```python
from build123d import *

# Parameters (mm, degrees)
SKETCH1_W           = 30
SKETCH1_H           = 13
BOSS_EXTRUDE1_DEPTH = 85
SKETCH2_W           = 22
SKETCH2_H           = 9
CUT_EXTRUDE2_DEPTH  = 85
SKETCH5_W           = 30
SKETCH5_H           = 13
BOSS_EXTRUDE3_DEPTH = 4
SKETCH12_W          = 22
SKETCH12_H          = 7
CUT_EXTRUDE4_DEPTH  = 13
SKETCH13_W          = 3
SKETCH13_H          = 80
CUT_EXTRUDE5_DEPTH  = 92.07140056


with BuildPart() as part:
    # Sketch1 → Boss-Extrude1 (new body)
    with BuildSketch(Plane(origin=(0, 0, 0), x_dir=(1, 0, 0), z_dir=(0, 1, 0))):
        with Locations((15, -6.5)):
            Rectangle(SKETCH1_W, SKETCH1_H)
    extrude(amount=BOSS_EXTRUDE1_DEPTH)

    # Sketch2 → Cut-Extrude2 (cut)
    with BuildSketch(Plane(origin=(0, 85, 0), x_dir=(1, 0, 0), z_dir=(0, 1, 0))):
        with Locations((15, -6.5)):
            Rectangle(SKETCH2_W, SKETCH2_H)
    extrude(amount=-CUT_EXTRUDE2_DEPTH, mode=Mode.SUBTRACT)

    # Sketch5 → Boss-Extrude3 (add)
    with BuildSketch(Plane(origin=(0, 0, 0), x_dir=(1, 0, 0), z_dir=(0, 1, 0))):
        with Locations((15, -6.5)):
            Rectangle(SKETCH5_W, SKETCH5_H)
    extrude(amount=-BOSS_EXTRUDE3_DEPTH)

    # Sketch12 → Cut-Extrude4 (cut)
    with BuildSketch(Plane.XY.offset(13)):
        with Locations((15, 3.5)):
            Rectangle(SKETCH12_W, SKETCH12_H)
    extrude(amount=-CUT_EXTRUDE4_DEPTH, mode=Mode.SUBTRACT)

    # Sketch13 → Cut-Extrude5 (cut, through all)
    with BuildSketch(Plane.ZY):
        with Locations((6.5, 40)):
            Rectangle(SKETCH13_W, SKETCH13_H)
    extrude(amount=-CUT_EXTRUDE5_DEPTH, mode=Mode.SUBTRACT)


solid = part.part
```
The model under review builds one solid part; all positions refer to its coordinate system, in mm. A direction names the side the tool comes from. Give positions to 0.01 mm unless a question says otherwise; leave off trailing zeros. Order: outer loops, then holes, each group sorted by start corner. A loop starts at its lowest first (then second) coordinate and runs counter-clockwise, first axis right, second up. Notation, with made-up numbers: (33, 83.25) - (52, 83.25) arc R18 ccw to (52, 115.25) - close; hole circle Ø3 at (81, -17.5). An arc over 180 degrees is marked (long way). Use CSV: the item, a comma, the result in double quotes. Start each with the question number.
Q1. We need section B-B, the plane x = 21.25. Write out the cut boundary in (y, z).
Q2. The part is to be moulded in two halves that separate along X. For faces 1 (the flat face through (0, 41, 9)), 2 (the flat face through (28, 39, 8)), 3 (the flat face through (15, 7, 1)), say which applies: +X half, -X half, draft (parallel to the pull), parting line (faces both ways), or undercut.
Q3. We need section C-C, the plane y = 16. Write out the cut boundary in (x, z), and give its area (3 significant figures).
Q4. To check wall thickness, follow line 1 along Y through (x, z) = (1.75, 7); line 2 along X through (y, z) = (25, 10.75); line 3 along Z through (x, y) = (26.75, 77). State the ranges of each line that lie inside material, in increasing order. Write a range as [from, to].
Q5. Tool access review of faces 4 (the flat face through (15, 47, 2)), 5 (the flat face through (28, 39, 5)), 6 (the flat face through (30, 41, 9)): name each direction out of +Z, -Z, +X, -X, +Y, -Y from which nothing blocks a thin tool from reaching the whole face with its end or side.
Q6. We need section A-A, the plane y = 5.5. Write out the cut boundary in (x, z), and give its area (3 significant figures).
Q7. We need section D-D, the plane z = 6.75. Write out the cut boundary in (x, y), and give its area (3 significant figures).
Outcome:
1,outline,"(-4, 0) - (0, 0) - (0, 13) - (-4, 13) - close; (7, 0) - (85, 0) - (85, 2) - (7, 2) - close; (7, 11) - (85, 11) - (85, 13) - (7, 13) - close"
2,face 1,"-X half"
2,face 2,"draft"
2,face 3,"undercut"
3,outline,"(0, 0) - (30, 0) - (30, 5) - (26, 5) - (26, 2) - (4, 2) - (4, 5) - (0, 5) - close; (0, 8) - (4, 8) - (4, 11) - (26, 11) - (26, 8) - (30, 8) - (30, 13) - (0, 13) - close"
3,area,"168 mm^2"
4,line 1,"y = [-4, 0], [80, 85]"
4,line 2,"x = [0, 4], [26, 30]"
4,line 3,"z = [0, 5], [8, 13]"
5,face 4,"+Y"
5,face 5,"+X, -X"
5,face 6,"+Z, -Z, +X, +Y, -Y"
6,outline,"(0, 0) - (4, 0) - (4, 5) - (0, 5) - close; (0, 8) - (4, 8) - (4, 13) - (0, 13) - close; (26, 0) - (30, 0) - (30, 5) - (26, 5) - close; (26, 8) - (30, 8) - (30, 13) - (26, 13) - close"
6,area,"80.0 mm^2"
7,outline,"(0, -4) - (30, -4) - (30, 0) - (0, 0) - close; (0, 80) - (4, 80) - (4, 85) - (0, 85) - close; (26, 80) - (30, 80) - (30, 85) - (26, 85) - close"
7,area,"160 mm^2"
